Design review of the part built by this model. Coordinates are the model's own, in mm. Face numbers are marked on the shaded views. Round coordinates to 2 decimals unless told otherwise and drop trailing zeros. Order: outer loops, then holes, each group sorted by start corner. A loop starts at its lowest first (then second) coordinate and runs counter-clockwise, first axis right, second up.
from build123d import *

# Parameters (mm, degrees)
F1_DEPTH = 300
F3_DEPTH = 300
F4_W     = 73.538634
F4_H     = 45.165462
F5_DEPTH = 300
F6_W     = 10.41078
F6_H     = 80
F7_DEPTH = 8


with BuildPart() as f1:
    # F0 (on Front) → F1 (new body)
    with BuildSketch(Plane.XZ):
        with BuildLine():
            ThreePointArc((0, 49.64232), (-18.760966, -5.35768), (0, -60.35768))
            ThreePointArc((0, -60.35768), (18.760966, -5.35768), (0, 49.64232))
        make_face()
    extrude(amount=F1_DEPTH)

    # F2 (on face) → F3 (cut)
    with BuildSketch(Plane.XZ.offset(300)):
        with BuildLine():
            ThreePointArc((0, 34.64232), (-15.27864, -5.35768), (0, -45.35768))
            ThreePointArc((0, -45.35768), (15.27864, -5.35768), (0, 34.64232))
        make_face()
    extrude(amount=-F3_DEPTH, mode=Mode.SUBTRACT)

    # F4 (on face) → F5 (cut)
    with BuildSketch(Plane.XZ.offset(300)):
        with Locations((-1.304593, 64.725051)):
            Rectangle(F4_W, F4_H)
    extrude(amount=-F5_DEPTH, mode=Mode.SUBTRACT)

    # F6 (on face) → F7 (cut)
    with BuildSketch(Plane.XY.offset(42.14232)):
        with Locations((0, -150)):
            Rectangle(F6_W, F6_H)
    extrude(amount=-F7_DEPTH, mode=Mode.SUBTRACT)


solid = f1.part
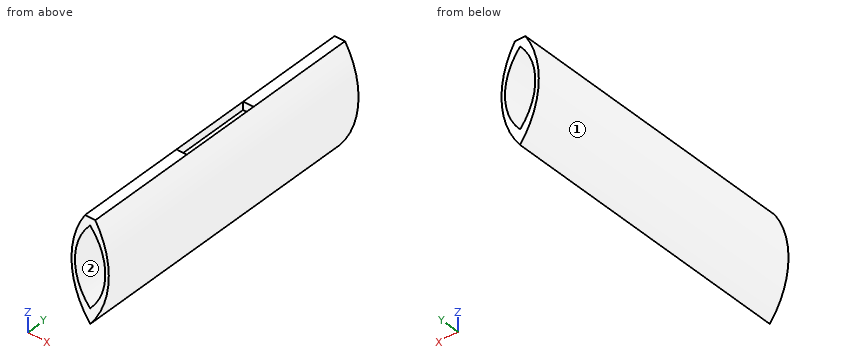
1) The part is to be moulded in two halves that separate along Z. For the marked faces 1 and 2, say which applies: released by +Z, released by -Z, zero draft, split by the parting line, or undercut.
Results:
face 1: split by the parting line
face 2: undercut
2) Clearance check with flat-ended pins moving along their axes: P1, Ø6, axis at y = -96.5, z = 4, coming from the +X side; P2, Ø2.5, axis at x = -2, y = -158, coming from the +Z side; P3, Ø5, axis at x = -12, y = -149.5, coming from the +Z side. State where each tip first meets the part, or that it passes through.
Results:
P1: stops at x = 18.54
P2: stops at z = 34.14
P3: stops at z = 34.41
3) Take a section at C-C on x = 12. Give the boundary of the cut face in (y, z), plus the area to 3 significant figures.
Results:
outline: (-300, -39.58) - (0, -39.58) - (0, -24.92) - (-300, -24.92) - close; (-300, 14.2) - (0, 14.2) - (0, 28.87) - (-300, 28.87) - close
area: 8,800 mm2
4) To check wall thickness, follow line 1 along X through (y, z) = (-34, -6.5); line 2 along X through (y, z) = (-162, -8); line 3 along Z through (x, y) = (7.5, -121). State the ranges of each line that lie inside material, in increasing order.
Results:
line 1: x = -18.75 to -15.27, 15.27 to 18.75
line 2: x = -18.72 to -15.22, 15.22 to 18.72
line 3: z = -48.95 to -34.9, 24.19 to 38.23
5) Take a section at A-A on z = 14.5. Give the boundary of the cut face in (x, y), plus the area to 3 significant figures.
Results:
outline: (-16.54, -300) - (-11.9, -300) - (-11.9, 0) - (-16.54, 0) - close; (11.9, -300) - (16.54, -300) - (16.54, 0) - (11.9, 0) - close
area: 2,790 mm2
6) Take a section at B-B on y = -38. Give the boundary of the cut face in (x, z), plus the area to 3 significant figures.
Results:
outline: (-5.21, 42.14) arc R90 ccw to (0, -60.36) arc R90 ccw to (5.21, 42.14) - close; hole (0, -45.36) arc R60 ccw to (0, 34.64) arc R60 ccw to start
area: 1,100 mm2
